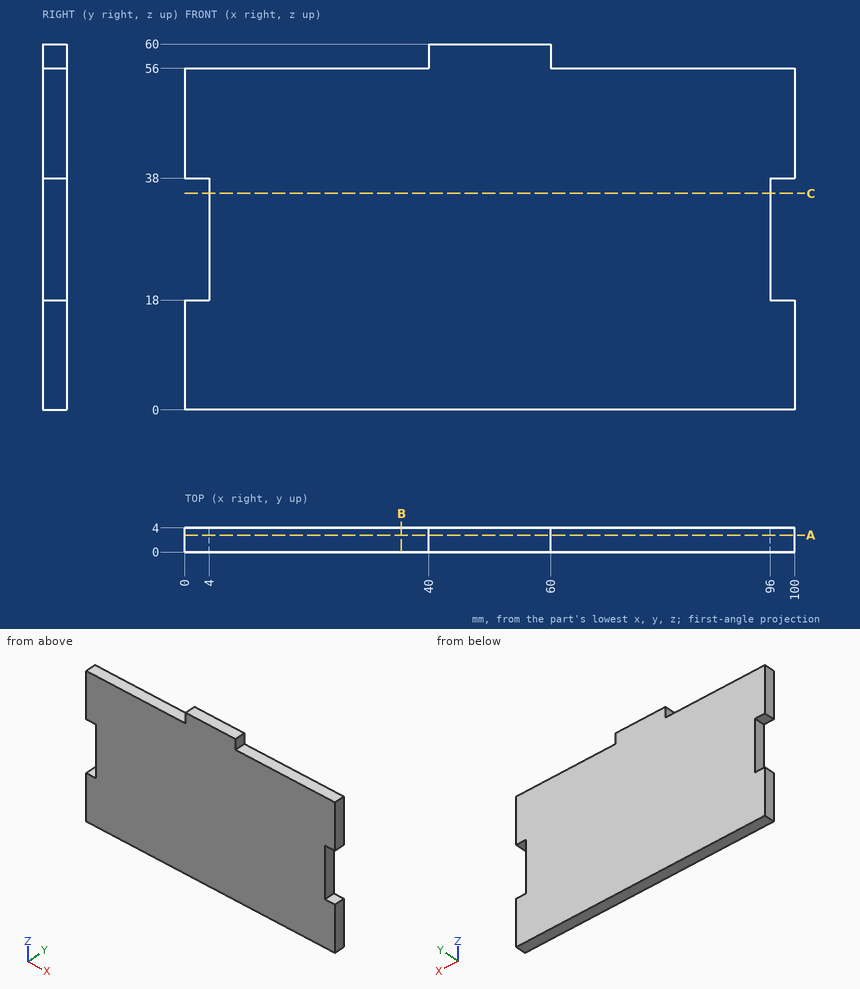
Can you work these out from the drawing? Everything is in mm from the part's minimum corner. Round coordinates to 2 decimals unless told otherwise and drop trailing zeros. Write each loop counter-clockwise with the first axis right and the second up, starting at its lowest first coordinate (ties: lowest second). Pieces come first, ordered by that corner, then holes. Notation, with made-up numbers: (62.5, 39) - (96.5, 39) arc R23 cw to (96.5, 67) - close; hole circle Ø7 at (45, -20.75). An arc over 180 degrees is marked (long way). Put each result on its own line as item: value. Start each with the question number.
(1) Will these pins go through, and if not, where does the flat tip stop? pin 1 (1.2 mm diameter, centred on y = 2, z = 30, fed in from +X); pin 2 (1.2 mm diameter, centred on x = 2, y = 1, fed in from +Z); pin 3 (1.2 mm diameter, centred on y = 2.5, z = 58, fed in from -X).
(2) I want a section at A-A, the plane y = 2.8. Please give me the cut outline in (x, z), plus the area to 3 significant figures.
(3) I want a section at B-B, the plane x = 35.5. Please give me the cut outline in (y, z).
(4) I need wall thicknesses on probe 1 along Z at (x, y) = (70, 3.35); probe 2 along X at (y, z) = (1.55, 22.5). Which ranges of each line are inside material? Lowest first, please.
(5) I want a section at C-C, the plane z = 35.5. Please give me the cut outline in (x, y).
Here are the results:
1. pin 1: stops at x = 96
1. pin 2: stops at z = 56
1. pin 3: stops at x = 40
2. outline: (0, 0) - (100, 0) - (100, 18) - (96, 18) - (96, 38) - (100, 38) - (100, 56) - (60, 56) - (60, 60) - (40, 60) - (40, 56) - (0, 56) - (0, 38) - (4, 38) - (4, 18) - (0, 18) - close
2. area: 5,520 mm^2
3. outline: (0, 0) - (4, 0) - (4, 56) - (0, 56) - close
4. probe 1: z = 0 to 56
4. probe 2: x = 4 to 96
5. outline: (4, 0) - (96, 0) - (96, 4) - (4, 4) - close
